```python
from build123d import *

# Parameters (mm, degrees)
F0_W      = 60
F0_H      = 90
F1_DEPTH  = 2
F2_W      = 22
F2_H      = 32
F3_DEPTH  = 1
F4_R      = 1.25
F5_DEPTH  = 1
F6_R      = 0.5
F7_DEPTH  = 1
F8_R      = 7.5
F9_R      = 7.5
F11_DEPTH = 2
F12_R     = 1.5
F13_DEPTH = 3
F14_W     = 3.5
F14_H     = 30
F15_DEPTH = 2
F16_W     = 21
F16_H     = 3.5
F17_DEPTH = 2
F18_W     = 21
F18_H     = 3.5
F19_DEPTH = 2
F20_R     = 1.25
F21_DEPTH = 25
F22_R     = 1.5
F23_DEPTH = 25


with BuildPart() as f1:
    # F0 (on Front) → F1 (new body)
    with BuildSketch(Plane.XZ):
        with Locations((30, 45)):
            Rectangle(F0_W, F0_H)
    extrude(amount=F1_DEPTH)

    # F2 (on face) → F3 (cut)
    with BuildSketch(Plane.XZ.offset(2)):
        with Locations((28.5, 44)):
            Rectangle(F2_W, F2_H)
    extrude(amount=-F3_DEPTH, mode=Mode.SUBTRACT)

    # F4 (on face) → F5 (join)
    with BuildSketch(Plane.XZ.offset(1)):
        with Locations((20.5, 53)):
            Circle(F4_R)
        with Locations((36.5, 33)):
            Circle(F4_R)
    extrude(amount=F5_DEPTH)

    # F6 (on face) → F7 (cut)
    with BuildSketch(Plane.XZ.offset(2)):
        with Locations((20.5, 53)):
            Circle(F6_R)
        with Locations((36.5, 33)):
            Circle(F6_R)
    extrude(amount=-F7_DEPTH, mode=Mode.SUBTRACT)

    # F8
    f8_edges = [f1.edges().sort_by_distance(p)[0] for p in [
        (60, -1, 90),
    ]]
    fillet(f8_edges, radius=F8_R)

    # F9
    f9_edges = [f1.edges().sort_by_distance(p)[0] for p in [
        (0, -1, 90),
        (0, -1, 0),
        (60, -1, 0),
    ]]
    fillet(f9_edges, radius=F9_R)

    # F10 (on face) → F11 (join)
    with BuildSketch(Plane.XZ.offset(2)):
        Polygon((0, 45), (0, 55), (-4, 52.5), (-4, 47.5), align=None)
        Polygon((64, 52.5), (60, 55), (60, 45), (64, 47.5), align=None)
        Polygon((27.5, 94), (25, 90), (35, 90), (32.5, 94), align=None)
        Polygon((35, 0), (25, 0), (27.5, -4), (32.5, -4), align=None)
    extrude(amount=-F11_DEPTH)

    # F12 (on face) → F13 (cut)
    with BuildSketch(Plane.XZ.offset(2)):
        with Locations((30, 91.85)):
            Circle(F12_R)
        with Locations((61.85, 50)):
            Circle(F12_R)
        with Locations((30, -1.85)):
            Circle(F12_R)
        with Locations((-1.85, 50)):
            Circle(F12_R)
    extrude(amount=-F13_DEPTH, mode=Mode.SUBTRACT)

    # F14 (on face) → F15 (join)
    with BuildSketch(Plane.XZ.offset(2)):
        with Locations((8.25, 45)):
            Rectangle(F14_W, F14_H)
        with Locations((48.75, 45)):
            Rectangle(F14_W, F14_H)
    extrude(amount=F15_DEPTH)

    # F16 (on face) → F17 (join)
    with BuildSketch(Plane.XZ.offset(2)):
        with Locations((30, 9.25)):
            Rectangle(F16_W, F16_H)
    extrude(amount=F17_DEPTH)

    # F18 (on face) → F19 (join)
    with BuildSketch(Plane.XZ.offset(2)):
        with Locations((30, 80.75)):
            Rectangle(F18_W, F18_H)
    extrude(amount=F19_DEPTH)

    # F20 (on face) → F21 (cut)
    with BuildSketch(Plane.XZ.offset(2)):
        with Locations((4.0452558799, 85.4404978659)):
            Circle(F20_R)
        with Locations((55.9547441201, 85.4404978659)):
            Circle(F20_R)
        with Locations((55.6786040567, 4.3146376432)):
            Circle(F20_R)
        with Locations((4.3180194842, 4.3180194851)):
            Circle(F20_R)
        with Locations((7.146446609, 7.1464466098)):
            Circle(F20_R)
        with Locations((52.8565831787, 7.1494565376)):
            Circle(F20_R)
        with Locations((52.3295245454, 83.75)):
            Circle(F20_R)
        with Locations((7.6704754546, 83.75)):
            Circle(F20_R)
    extrude(amount=-F21_DEPTH, mode=Mode.SUBTRACT)

    # F22 (on face) → F23 (cut)
    with BuildSketch(Plane.XZ.offset(2)):
        with Locations((5, 72.5)):
            Circle(F22_R)
        with Locations((5, 17.5)):
            Circle(F22_R)
        with Locations((55, 72.5)):
            Circle(F22_R)
        with Locations((55, 17.5)):
            Circle(F22_R)
    extrude(amount=-F23_DEPTH, mode=Mode.SUBTRACT)


solid = f1.part
```
Work out the finished part from the listing and answer in its coordinate system (mm). A direction names the side the tool comes from. Give positions to 0.01 mm unless a question says otherwise; leave off trailing zeros. Loops run counter-clockwise (first coordinate to the right, second up) from the corner with the lowest first, then second, coordinate; pieces in that order, holes last. Notation, with made-up numbers: M -4,32.25 L 30,32.25 A24 cw 30,55.25 Z; hole C 66,23 d8. An arc over 180 degrees is marked long. One line per item, written item: value. Start each with the question number.
1. Find section C-C (x = 61.85). Give the vertices of the cut face in (y, z), and give its area (4 significant figures).
2. Find the intervals of material crossed by probe 1 along Z at (x, y) = (30, -0.7); probe 2 along Z at (x, y) = (30, -1.2); probe 3 along X at (y, z) = (-3.3, 55), in increasing order.
3. Determine the mould class of faces 5 (the face through (44, -1, 0)), 6 (the face through (2.255, -1.014, 87.861)), 7 (the face through (19.5, -3, 81)), 8 (the face through (45, -2, 46)) for opening direction Z: released by +Z, released by -Z, zero draft, split by the parting line, or undercut.
4. Find section B-B (y = -2.8). Give the vertices of the cut face in (x, z).
5. Each of these flat-tipped pins is pushed along its axis until it touches: P1, Ø1.1, axis at x = 36.5, z = 33, coming from the -Y side; P2, Ø0.6, axis at x = 31, y = -3, coming from the -Z side; P3, Ø0.6, axis at x = 32.5, y = -3, coming from the +Z side; P4, Ø2, axis at x = 4.05, z = 85.44, coming from the -Y side. Where does it stop, or does it pass through?
6. Find section A-A (z = 50). Give the vertices of the cut face in (x, y), and give its area (3 significant figures).
7. Which of the six approach directions +Z, -Z, +X, -X, +Y, -Y give full straight-line access (tool end or side, diameter ignored) to faces 1 (the face through (0, -1, 69)), 2 (the face through (30, -3, 7.5)), 3 (the face through (35.25, -1.49, 33.05)), 4 (the face through (60, -1, 69))?
8. Find section D-D (z = -1.85). Give the vertices of the cut face in (x, y).
Reported:
1. outline: M -2,46.16 L 0,46.16 L 0,48.5 L -2,48.5 Z; M -2,51.5 L 0,51.5 L 0,53.84 L -2,53.84 Z
1. area: 9.375 mm²
2. probe 1: z = -4 to -3.35, -0.35 to 90.35, 93.35 to 94
2. probe 2: z = -4 to -3.35, -0.35 to 28, 60 to 90.35, 93.35 to 94
2. probe 3: x = 6.5 to 10, 47 to 50.5
3. face 5: released by -Z
3. face 6: released by +Z
3. face 7: zero draft
3. face 8: undercut
4. outline: M 6.5,30 L 10,30 L 10,60 L 6.5,60 Z; M 19.5,7.5 L 40.5,7.5 L 40.5,11 L 19.5,11 Z; M 19.5,79 L 40.5,79 L 40.5,82.5 L 19.5,82.5 Z; M 47,30 L 50.5,30 L 50.5,60 L 47,60 Z
5. P1: stops at y = -2
5. P2: stops at z = 7.5
5. P3: stops at z = 82.5
5. P4: passes through
6. outline: M -4,-2 L -3.35,-2 L -3.35,0 L -4,0 Z; M -0.35,-2 L 6.5,-2 L 6.5,-4 L 10,-4 L 10,-2 L 17.5,-2 L 17.5,-1 L 39.5,-1 L 39.5,-2 L 47,-2 L 47,-4 L 50.5,-4 L 50.5,-2 L 60.35,-2 L 60.35,0 L -0.35,0 Z; M 63.35,-2 L 64,-2 L 64,0 L 63.35,0 Z
6. area: 116 mm²
7. face 1: +Z, -X, +Y, -Y
7. face 2: -Z, +X, -X, -Y
7. face 3: -Y
7. face 4: +Z, +X, +Y, -Y
8. outline: M 26.16,-2 L 28.5,-2 L 28.5,0 L 26.16,0 Z; M 31.5,-2 L 33.84,-2 L 33.84,0 L 31.5,0 Z
